```python
from build123d import *

# Parameters (mm, degrees)
F0_W     = 80
F0_H     = 15
F1_DEPTH = 8
F2_W     = 80
F2_H     = 5.823
F3_DEPTH = 25
F4_DEPTH = 7


with BuildPart() as f1:
    # F0 (on Top) → F1 (new body)
    with BuildSketch(Plane.XY):
        with Locations((17.0978596434, -1.9628690071)):
            Rectangle(F0_W, F0_H)
    extrude(amount=F1_DEPTH)

    # F2 (on face) → F3 (join)
    with BuildSketch(Plane.XY.offset(8)):
        with Locations((17.0978596434, -6.5513690071)):
            Rectangle(F2_W, F2_H)
    extrude(amount=F3_DEPTH)

    # F4 (add): a face of the model
    f4_faces = [f1.faces().sort_by_distance(p)[0] for p in [
        (17.0978596434, 5.5371309929, 4),
    ]]
    extrude(f4_faces, amount=F4_DEPTH)


solid = f1.part
```
CAD build for the part. Positions are in the model's coordinates, mm. A direction names the side the tool comes from. Round coordinates to 2 decimals unless told otherwise and drop trailing zeros. Order: outer loops, then holes, each group sorted by start corner. A loop starts at its lowest first (then second) coordinate and runs counter-clockwise, first axis right, second up.
Item 1: Pin check, flat tip, straight feed: pin 1 (3 mm diameter, centred on x = -8.5, y = 10, fed in from +Z). Stop position of the tip, or through.
Item 2: Saw through at B-B on x = -15.5. Write the cut outline in (y, z).
Item 3: Saw through at A-A on y = 10.25. Write the cut outline in (x, z), then the cut area to 3 significant figures.
Item 4: Saw through at C-C on z = 16.5. Write the cut outline in (x, y).
Item 5: Probe line 1 along Z through (x, y) = (12, 8); line 2 along Y through (x, z) = (13, 11). List the from-to ranges inside material, lowest first.
Item 6: Tool access for faces 1 (the face through (17, 4, 8)), 2 (the face through (17, -9.463, 16)): list every direction of +Z, -Z, +X, -X, +Y, -Y with a clear straight run to the whole face (end or side of a thin tool).
Reported:
1. pin 1: stops at z = 8
2. outline: (-9.46, 0) - (12.54, 0) - (12.54, 8) - (-3.64, 8) - (-3.64, 33) - (-9.46, 33) - close
3. outline: (-22.9, 0) - (57.1, 0) - (57.1, 8) - (-22.9, 8) - close
3. area: 640 mm2
4. outline: (-22.9, -9.46) - (57.1, -9.46) - (57.1, -3.64) - (-22.9, -3.64) - close
5. line 1: z = 0 to 8
5. line 2: y = -9.46 to -3.64
6. face 1: +Z, +X, -X, +Y
6. face 2: +Z, -Z, +X, -X, -Y
